from build123d import *

# Parameters (mm, degrees)
SKETCH1_W           = 150
SKETCH1_H           = 40.85
BOSS_EXTRUDE1_DEPTH = 3
SKETCH2_W           = 150
SKETCH2_H           = 3
BOSS_EXTRUDE2_DEPTH = 25
BOSS_EXTRUDE3_DEPTH = 150
SKETCH6_R           = 2.5
CUT_EXTRUDE2_DEPTH  = 10
SKETCH7_R           = 2.5
CUT_EXTRUDE3_DEPTH  = 160.045661682


with BuildPart() as part:
    # Sketch1 → Boss-Extrude1 (new body)
    with BuildSketch(Plane(origin=(0, 0, 0), x_dir=(1, 0, 0), z_dir=(0, 1, 0))):
        with Locations((-75, 20.425)):
            Rectangle(SKETCH1_W, SKETCH1_H)
    extrude(amount=BOSS_EXTRUDE1_DEPTH)

    # Sketch2 → Boss-Extrude2 (add)
    with BuildSketch(Plane(origin=(0, 3, 0), x_dir=(1, 0, 0), z_dir=(0, 1, 0))):
        with Locations((-75, 39.35)):
            Rectangle(SKETCH2_W, SKETCH2_H)
        with Locations((-75, 1.5)):
            Rectangle(SKETCH2_W, SKETCH2_H)
    extrude(amount=BOSS_EXTRUDE2_DEPTH)

    # Sketch5 → Boss-Extrude3 (add)
    with BuildSketch(Plane(origin=(0, 0, 0), x_dir=(0, 0, -1), z_dir=(1, 0, 0))):
        Polygon((3, 28), (-2, 28), (-2, -2), (42.85, -2), (42.85, 28), (37.85, 28), (37.85, 3), (3, 3), align=None)
    extrude(amount=-BOSS_EXTRUDE3_DEPTH)

    # Sketch6 → Cut-Extrude2 (cut)
    with BuildSketch(Plane(origin=(0, 3, 0), x_dir=(1, 0, 0), z_dir=(0, 1, 0))):
        with Locations(Location((-140, 20.425, 0), (0, 0, 270))):
            Circle(SKETCH6_R)
        with Locations(Location((-10, 20.425, 0), (0, 0, 270))):
            Circle(SKETCH6_R)
    extrude(amount=-CUT_EXTRUDE2_DEPTH, mode=Mode.SUBTRACT)

    # Sketch7 → Cut-Extrude3 (cut, through all)
    with BuildSketch(Plane.XY.offset(2)):
        with Locations((-142.5, 20.5)):
            Circle(SKETCH7_R)
        with Locations((-7.5, 20.5)):
            Circle(SKETCH7_R)
    extrude(amount=-CUT_EXTRUDE3_DEPTH, mode=Mode.SUBTRACT)


solid = part.part
Verification items for the finished model (mm, model axes). A direction names the side the tool comes from. Coordinates: 2 decimals unless noted, no trailing zeros. Order: outer loops, then holes, each group sorted by start corner. A loop starts at its lowest first (then second) coordinate and runs counter-clockwise, first axis right, second up. Notation, with made-up numbers: M -12.5,-11.5 L -6.5,-11.5 A33 cw -6.5,20.5 Z; hole C -18.75,50 d11. An arc over 180 degrees is marked long. One line per item, written item: value. Start each with the question number.
Item 1: Sectioned sample at D-D (z = -13). Enter the section's corners in (x, y).
Item 2: Scan lines: probe 1 along Z at (x, y) = (-25, 17); probe 2 along Y at (x, z) = (-142.5, 0.3); probe 3 along Z at (x, y) = (-140, 0.3) (3 decimals). Record each from-to range of solid material in increasing order.
Item 3: Sectioned sample at C-C (x = -14). Enter the section's corners in (y, z).
Item 4: Gauge pin test, flat end, axial feed: pin 1 (2 mm diameter, centred on x = -30.5, z = -35, fed in from +Y). Record the tip position at first contact, or that the pin passes through.
Item 5: Sectioned sample at A-A (y = 20.5). Enter the section's corners in (x, z), then the cut area to 3 significant figures.
Item 6: Mould release check, pull along Z, two halves, no side actions. Record for faces 1 (the flat face through (-74, -2, -20)), 2 (the flat face through (-74, 13, 2)), 3 (the cylindrical face through (-137.52, 0.54, -20.75)): released by +Z, released by -Z, zero draft, split by the parting line, or undercut.
Item 7: Access from +Z, -Z, +X, -X, +Y, -Y to the whole of each face (thin tool, end or side, straight path). Record for faces 4 (the cylindrical face through (-12.44, 0.54, -20.97)), 5 (the flat face through (-76, 15, -37.85)).
Item 8: Sectioned sample at B-B (y = 4.75). Enter the section's corners in (x, z), then the cut area to 3 significant figures.
Conclusion:
1. outline: M -150,-2 L 0,-2 L 0,3 L -150,3 Z
2. probe 1: z = -42.85 to -37.85, -3 to 2
2. probe 2: y = -2 to 18, 23 to 28
2. probe 3: z = -42.85 to -22.925, -17.925 to 2
3. outline: M -2,-42.85 L 28,-42.85 L 28,-37.85 L 3,-37.85 L 3,-3 L 28,-3 L 28,2 L -2,2 Z
4. pin 1: stops at y = 3
5. outline: M -150,-42.85 L -145,-42.85 L -145,-37.85 L -150,-37.85 Z; M -150,-3 L -145,-3 L -145,2 L -150,2 Z; M -140,-42.85 L -10,-42.85 L -10,-37.85 L -140,-37.85 Z; M -140,-3 L -10,-3 L -10,2 L -140,2 Z; M -5,-42.85 L 0,-42.85 L 0,-37.85 L -5,-37.85 Z; M -5,-3 L 0,-3 L 0,2 L -5,2 Z
5. area: 1,400 mm^2
6. face 1: zero draft
6. face 2: released by +Z
6. face 3: undercut
7. face 4: +Y, -Y
7. face 5: +X, -X, +Y
8. outline: M -150,-42.85 L 0,-42.85 L 0,-37.85 L -150,-37.85 Z; M -150,-3 L 0,-3 L 0,2 L -150,2 Z
8. area: 1,500 mm^2
